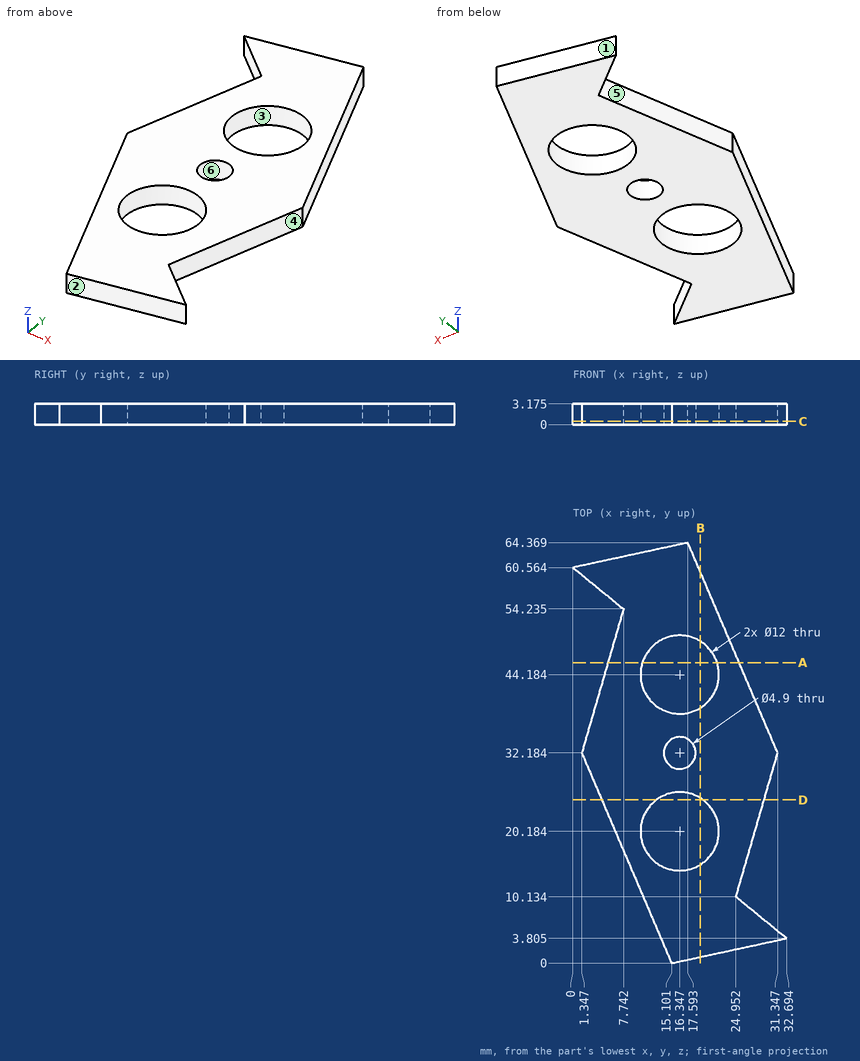
Check sheet for the drawn part. Datum: minimum x, y, z corner. Units: mm. A direction names the side the tool comes from. Round coordinates to 2 decimals unless told otherwise and drop trailing zeros. Order: outer loops, then holes, each group sorted by start corner. A loop starts at its lowest first (then second) coordinate and runs counter-clockwise, first axis right, second up. Notation, with made-up numbers: (-8, -33) - (28, -33) arc R23 cw to (28, 5) - close; hole circle Ø2 at (38.25, 8.25). An arc over 180 degrees is marked (long way). Use a Markdown table: item, result. Add a question column.
(1) Sectioned sample at C-C, the plane z = 0.5. Count the separate pieces of the cut face and the enclosed holes in it, and give its area (3 significant figures).
(2) Material ranges on line 1 along Y through (x, z) = (20, 2.2) (1 decimal); line 2 along Y through (x, z) = (21.5, 0.95) (1 decimal); line 3 along X through (y, z) = (16, 2.3) (1 decimal), recorded low to high. Write a range as [from, to].
(3) Sectioned sample at A-A, the plane y = 46. Enter the section's corners in (x, z) (1 decimal).
(4) Sectioned sample at D-D, the plane y = 25. Enter the section's corners in (x, z) (1 decimal).
(5) Tool access check on the marked faces 4, 5 and 6. Record the directions out of +Z, -Z, +X, -X, +Y, -Y that give a thin tool (end or side, any length) a straight path to the whole face; none if there is none.
(6) Release check for a two-part mould opening along Y. For the marked faces 1, 2 and 3 record: pulls with the +Y half, pulls with the -Y half, needs draft (parallel to the pull), parting line crosses it, or undercut.
(7) Depth check by flat-ended pin: pin 1 (15.5 mm diameter, centred on x = 16.35, y = 44.18, fed in from +Z) (3 decimals). Enter the tip coordinate at first touch or a pass-through.
(8) Sectioned sample at B-B, the plane x = 19.5. Enter the section's corners in (y, z) (1 decimal), and give its area (3 significant figures).
Answers below:
| question | item | result |
|---|---|---|
| 1 | separate pieces | 1 |
| 1 | enclosed holes | 3 |
| 1 | area | 1,010 mm² |
| 2 | line 1 | [1.1, 15.4], [24.9, 39.4], [48.9, 58.7] |
| 2 | line 2 | [1.4, 17.1], [23.3, 41.1], [47.3, 55.2] |
| 2 | line 3 | [8.3, 12], [20.6, 26.7] |
| 3 | outline | (5.4, 0) - (10.6, 0) - (10.6, 3.2) - (5.4, 3.2) - close; (22.1, 0) - (25.4, 0) - (25.4, 3.2) - (22.1, 3.2) - close |
| 4 | outline | (4.4, 0) - (12.8, 0) - (12.8, 3.2) - (4.4, 3.2) - close; (19.9, 0) - (29.3, 0) - (29.3, 3.2) - (19.9, 3.2) - close |
| 5 | face 4 | +Z, -Z, +X |
| 5 | face 5 | +Z, -Z, -X |
| 5 | face 6 | +Z, -Z |
| 6 | face 1 | pulls with the +Y half |
| 6 | face 2 | pulls with the -Y half |
| 6 | face 3 | undercut |
| 7 | pin 1 | z = 3.175 |
| 8 | outline | (1, 0) - (15.1, 0) - (15.1, 3.2) - (1, 3.2) - close; (25.3, 0) - (39.1, 0) - (39.1, 3.2) - (25.3, 3.2) - close; (49.3, 0) - (59.9, 0) - (59.9, 3.2) - (49.3, 3.2) - close |
| 8 | area | 122 mm² |
